Autodesk Inventor part; units mm, degrees
ref_plane "YZ Plane" through (0, 0, 0) normal (1, 0, 0) x (0, 1, 0)
ref_plane "XZ Plane" through (0, 0, 0) normal (0, 1, 0) x (-1, 0, 0)
ref_plane "XY Plane" through (0, 0, 0) normal (0, 0, 1) x (1, 0, 0)
ref_plane "Arbeitsebene1" through (63.727, -21.9316, 9.2792) normal (0, -1, 0) x (1, 0, 0)
sketch "Skizze1" plane through (63.727, -21.9316, 9.2792) normal (0, -1, 0) x (1, 0, 0)
  line L0 (-20.15, -16.7358) -> (-16.7358, -20.15)
  line L1 (-16.7358, -20.15) -> (16.7358, -20.15)
  line L2 (16.7358, -20.15) -> (20.15, -16.7358)
  line L3 (20.15, -16.7358) -> (20.15, 16.7358)
  line L4 (20.15, 16.7358) -> (16.7358, 20.15)
  line L5 (16.7358, 20.15) -> (-16.7358, 20.15)
  line L6 (-16.7358, 20.15) -> (-20.15, 16.7358)
  line L7 (-20.15, 16.7358) -> (-20.15, -16.7358)
  circle A0 centre (-15.5, -15.5) radius 2
  circle A1 centre (15.5, -15.5) radius 2
  circle A2 centre (15.5, 15.5) radius 2
  circle A3 centre (-15.5, 15.5) radius 2
  circle A4 centre (0, 0) radius 11.5
  line L8 (24.5, -28.5) -> (-24.5, -28.5)
  line L9 (-28.5, -24.5) -> (-28.5, 24.5)
  line L10 (-24.5, 28.5) -> (24.5, 28.5)
  line L11 (28.5, 24.5) -> (28.5, -24.5)
  line L12 (28.5, -28.5) -> (-28.5, 28.5) construction
  line L13 (-28.5, -28.5) -> (28.5, 28.5) construction
  arc A5 (-24.5, 28.5) -> (-28.5, 24.5) centre (-24.5, 24.5) ccw
  arc A6 (28.5, 24.5) -> (24.5, 28.5) centre (24.5, 24.5) ccw
  arc A7 (24.5, -28.5) -> (28.5, -24.5) centre (24.5, -24.5) ccw
  arc A8 (-28.5, -24.5) -> (-24.5, -28.5) centre (-24.5, -24.5) ccw
  line L14 (23.5, -23.5) -> (-23.5, -23.5) construction
  line L15 (-23.5, -23.5) -> (-23.5, 23.5) construction
  line L16 (-23.5, 23.5) -> (23.5, 23.5) construction
  line L17 (23.5, 23.5) -> (23.5, -23.5) construction
  line L18 (23.5, -23.5) -> (-23.5, 23.5) construction
  line L19 (-23.5, -23.5) -> (23.5, 23.5) construction
  circle A9 centre (-23.5, 23.5) radius 2
  circle A10 centre (23.5, 23.5) radius 2
  circle A11 centre (23.5, -23.5) radius 2
  circle A12 centre (-23.5, -23.5) radius 2
  point P0 (-63.727, -9.2792)
  dimension "d0" = 57
  dimension "d1" = 57
  dimension "d2" = 4
  dimension "d3" = 47
  dimension "d4" = 47
  dimension "d5" = 4
  dimension "d6" = 4
  dimension "d7" = 4
  dimension "d8" = 4
extrude "Extrusion1" add sketch "Skizze1" along normal blind 23 contours L7 L6 L5 L4 L3 L2 L1 L0 | L8 A8 L9 A5 L10 A6 L11 A7
properties part number "00_NEMA17_Perestalticpump_Adapter"
Check sheet for the modelled part. Datum: model origin and axes. Units: mm. Give positions to 0.01 mm unless a question says otherwise; leave off trailing zeros. Loops run counter-clockwise (first coordinate to the right, second up) from the corner with the lowest first, then second, coordinate; pieces in that order, holes last. Notation, with made-up numbers: M 58,-14 L 95,-14 A22 ccw 95,-4 Z; hole C -14.75,-25.5 d1. An arc over 180 degrees is marked long. Answer as a JSON object with one key per item and string values. Group by question number.
Q1. Cross-section at A-A on z = 7. Record the cut outline in (x, y), then the cut area to 3 significant figures.
Q2. Go/stop test with a flat-tipped pin: P1, Ø3, axis at x = 40.23, z = 32.78, coming from the -Y side. Record where the tip stops, or that it passes through.
Q3. Cross-section at C-C on z = -13.5. Record the cut outline in (x, y), then the cut area to 3 significant figures.
Q4. Release check for a two-part mould opening along X. For faces 1 (the flat face through (35.227, -33, 9)), 2 (the flat face through (64, -33, -19.221)), 3 (the cylindrical face through (41.15, -33.271, 34.554)), 4 (the cylindrical face through (91.02, -33.27, 36.64)) record: released by +X, released by -X, zero draft, split by the parting line, or undercut.
Q5. Cross-section at B-B on x = 54.5. Record the cut outline in (y, z).
Q6. Material ranges on line 1 along Z through (x, y) = (87, -41.5); line 2 along Z through (x, y) = (63.5, -34.5); line 3 along X through (y, z) = (-30, 32), recorded low to high. Write a range as [from, to].
Q7. Cross-section at D-D on y = -42. Give the number of separate pieces and of enclosed holes in the cut face, then the cut area to 3 significant figures.
Evaluation:
{
 "1": {"outline": "M 35.23,-44.93 L 52.46,-44.93 L 52.46,-21.93 L 35.23,-21.93 Z; M 75,-44.93 L 92.23,-44.93 L 92.23,-21.93 L 75,-21.93 Z", "area": "792 mm2"},
 "2": {"P1": "passes through"},
 "3": {"outline": "M 35.23,-44.93 L 38.36,-44.93 L 38.36,-21.93 L 35.23,-21.93 Z; M 42.09,-44.93 L 85.36,-44.93 L 85.36,-21.93 L 42.09,-21.93 Z; M 89.09,-44.93 L 92.23,-44.93 L 92.23,-21.93 L 89.09,-21.93 Z", "area": "1,140 mm2"},
 "4": {"face 1": "released by -X", "face 2": "zero draft", "face 3": "undercut", "face 4": "released by +X"},
 "5": {"outline": "M -44.93,-19.22 L -21.93,-19.22 L -21.93,2.42 L -44.93,2.42 Z; M -44.93,16.14 L -21.93,16.14 L -21.93,37.78 L -44.93,37.78 Z"},
 "6": {"line 1": "z = [-19.22, -16.21], [-12.23, 30.79], [34.77, 37.78]", "line 2": "z = [-19.22, -2.22], [20.78, 37.78]", "line 3": "x = [35.23, 38.39], [42.07, 85.39], [89.07, 92.23]"},
 "7": {"separate pieces": "1", "enclosed holes": "9", "area": "2,720 mm2"}
}
